```python
from build123d import *

# Parameters (mm, degrees)
SKETCH_2_W          = 30
SKETCH_2_H          = 30
SKETCH_2_R          = 5
EXTRUDE_1_DEPTH     = 4.5
CUT_EXTRUDE_1_DEPTH = 35.5325933
CUT_EXTRUDE_2_DEPTH = 8


with BuildPart() as part:
    # 草图2 → 凸台-拉伸1 (new body)
    with BuildSketch(Plane.XY):
        with Locations((0, 1.5)):
            Rectangle(SKETCH_2_W, SKETCH_2_H)
        with Locations((0, -6)):
            Circle(SKETCH_2_R, mode=Mode.SUBTRACT)
    extrude(amount=EXTRUDE_1_DEPTH)

    # 草图4 → 切除-拉伸1 (cut, through all)
    with BuildSketch(Plane(origin=(15, 0, 0), x_dir=(0, 0, -1), z_dir=(1, 0, 0))):
        with BuildLine():
            Line((-4.5, 7.5), (-3.82, 7.5))
            ThreePointArc((-3.82, 7.5), (-3.408962817, 7.219957697), (-2.941534065, 7.05))
            Line((-2.941534065, 7.05), (-1.7, 7.05))
            Line((-1.7, 7.05), (-1.7, 10.95))
            Line((-1.7, 10.95), (-2.941534065, 10.95))
            ThreePointArc((-2.941534065, 10.95), (-3.408962817, 10.780042303), (-3.82, 10.5))
            Line((-3.82, 10.5), (-4.5, 10.5))
            Line((-4.5, 10.5), (-4.5, 7.5))
        make_face()
    extrude(amount=-CUT_EXTRUDE_1_DEPTH, mode=Mode.SUBTRACT)

    # 草图5 → 切除-拉伸2 (cut)
    with BuildSketch(Plane(origin=(15, 0, 0), x_dir=(0, 0, -1), z_dir=(1, 0, 0))):
        with BuildLine():
            Line((-1.7, -4.05), (-1.7, -7.95))
            Line((-1.7, -7.95), (-2.941534065, -7.95))
            ThreePointArc((-2.941534065, -7.95), (-3.408962817, -7.780042303), (-3.82, -7.5))
            Line((-3.82, -7.5), (-4.5, -7.5))
            Line((-4.5, -7.5), (-4.5, -4.5))
            Line((-4.5, -4.5), (-3.82, -4.5))
            ThreePointArc((-3.82, -4.5), (-3.408962817, -4.219957697), (-2.941534065, -4.05))
            Line((-2.941534065, -4.05), (-1.7, -4.05))
        make_face()
    cut_extrude_2 = extrude(amount=-CUT_EXTRUDE_2_DEPTH, mode=Mode.SUBTRACT)

    # 镜向1: 切除-拉伸2 across plane
    add(cut_extrude_2.mirror(Plane(origin=(0, 0, 0), x_dir=(0, 0, 1), z_dir=(1, 0, 0))), mode=Mode.SUBTRACT)


solid = part.part
```
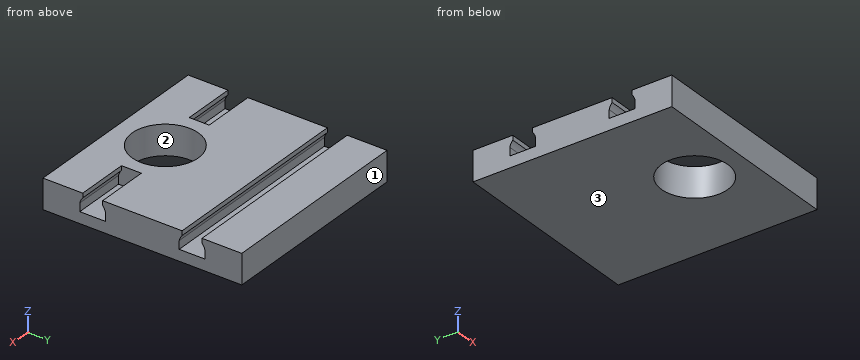
Read the model definition and answer for the solid it produces. Units are mm, in the model's axes. Face numbers are marked on the shaded views. Give positions to 0.01 mm unless a question says otherwise; leave off trailing zeros. Order: outer loops, then holes, each group sorted by start corner. A loop starts at its lowest first (then second) coordinate and runs counter-clockwise, first axis right, second up. Notation, with made-up numbers: (61, 33.5) -> (101, 33.5) arc R23 ccw to (101, 70.5) -> close; hole circle Ø10 at (68, 7.5). An arc over 180 degrees is marked (long way). Write item = value, one per line.
1. A cutting plane is placed at D-D, the plane x = 6.5. Write down the section's boundary in (y, z), and give its area (3 significant figures).
Numbers:
outline = (-13.5, 0) -> (16.5, 0) -> (16.5, 4.5) -> (10.5, 4.5) -> (10.5, 3.82) arc R2 cw to (10.95, 2.94) -> (10.95, 1.7) -> (7.05, 1.7) -> (7.05, 2.94) arc R2 cw to (7.5, 3.82) -> (7.5, 4.5) -> (-13.5, 4.5) -> close
area = 125 mm²
2. A cutting plane is placed at A-A, the plane y = -6. Write down the section's boundary in (x, z), and give its area (3 significant figures).
Numbers:
outline = (-15, 0) -> (-5, 0) -> (-5, 4.5) -> (-7, 4.5) -> (-7, 1.7) -> (-15, 1.7) -> close; (5, 0) -> (15, 0) -> (15, 1.7) -> (7, 1.7) -> (7, 4.5) -> (5, 4.5) -> close
area = 45.2 mm²
3. Given pin 1 (2 mm diameter, centred on y = -6.5, z = 2.5, fed in from -X); pin 2 (1 mm diameter, centred on x = 4.5, y = 8.5, fed in from +Z); pin 3 (0.8 mm diameter, centred on y = -5.5, z = 3, fed in from +X); pin 4 (1.4 mm diameter, centred on y = -6.5, z = 3.5, fed in from -X), each flat-ended and moving along its own axis, determine where each tip first touches the part or whether it passes through.
Numbers:
pin_1 = -15
pin_2 = 1.7
pin_3 = 7
pin_4 = -7
4. The mould has two halves that part along Y. Classify the marked faces 1, 2 and 3: +Y half, -Y half, draft (parallel to the pull), parting line (faces both ways), or undercut.
Numbers:
face_1 = +Y half
face_2 = undercut
face_3 = draft
5. A cutting plane is placed at C-C, the plane z = 0.5. Write down the section's boundary in (x, y).
Numbers:
outline = (-15, -13.5) -> (15, -13.5) -> (15, 16.5) -> (-15, 16.5) -> close; hole circle Ø10 at (0, -6)
6. Straight lines are drawn through the part: line 1 along Y through (x, z) = (0, 2.6); line 2 along Y through (x, z) = (0, 1.1); line 3 along Y through (x, z) = (9.75, 4.1). For each, find the intervals that lie inside material, in ascending order.
Numbers:
line_1 = -13.5 to -11, -1 to 7.05, 10.95 to 16.5
line_2 = -13.5 to -11, -1 to 16.5
line_3 = -13.5 to -7.5, -4.5 to 7.5, 10.5 to 16.5
7. A cutting plane is placed at B-B, the plane x = 0. Write down the section's boundary in (y, z), and give its area (3 significant figures).
Numbers:
outline = (-13.5, 0) -> (-11, 0) -> (-11, 4.5) -> (-13.5, 4.5) -> close; (-1, 0) -> (16.5, 0) -> (16.5, 4.5) -> (10.5, 4.5) -> (10.5, 3.82) arc R2 cw to (10.95, 2.94) -> (10.95, 1.7) -> (7.05, 1.7) -> (7.05, 2.94) arc R2 cw to (7.5, 3.82) -> (7.5, 4.5) -> (-1, 4.5) -> close
area = 80.0 mm²
